Model file for the job. Use its own axes, mm. Coordinates: 2 decimals unless noted, no trailing zeros. Write each loop counter-clockwise with the first axis right and the second up, starting at its lowest first coordinate (ties: lowest second). Pieces come first, ordered by that corner, then holes. Notation, with made-up numbers: M 27,52 L 74,52 A33 cw 74,80 Z; hole C -35.5,12 d5. An arc over 180 degrees is marked long. Use CSV: the item, a comma, the result in double quotes. Start each with the question number.
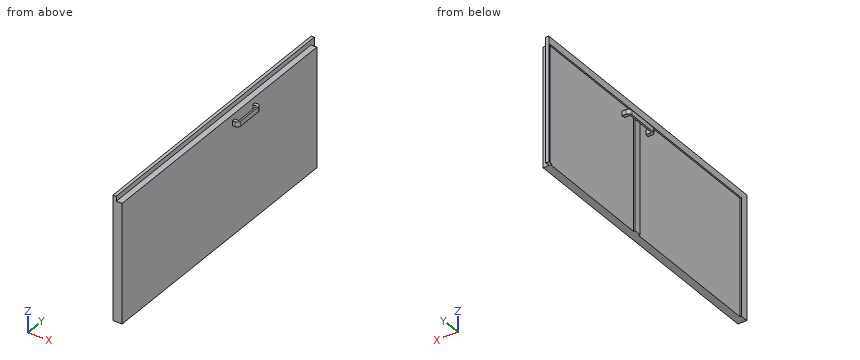
from build123d import *

# Parameters (mm, degrees)
SKETCH1_W            = 54.758446478
SKETCH1_H            = 717
BOSS_EXTRUDE1_DEPTH  = 1725
SKETCH2_W            = 19.21757675
SKETCH2_H            = 1725
BOSS_EXTRUDE2_DEPTH  = 30
SKETCH3_W            = 19.21757675
SKETCH3_H            = 747.470855808
BOSS_EXTRUDE3_DEPTH  = 30
SKETCH5_W            = 704.182305872
SKETCH5_H            = 1697.425748722
CUT_EXTRUDE1_DEPTH   = 8.60534571
SKETCH6_W            = 704.182305872
SKETCH6_H            = 43.914333375
BOSS_EXTRUDE5_DEPTH  = 9
SKETCH7_W            = 29.914870165
SKETCH7_H            = 20.630944942
BOSS_EXTRUDE6_DEPTH  = 35
SKETCH8_W            = 29.914870164
SKETCH8_H            = 20.630944941
BOSS_EXTRUDE7_DEPTH  = 35
SKETCH9_W            = 27.336002047
SKETCH9_H            = 231.066583342
BOSS_EXTRUDE8_DEPTH  = 10
SKETCH10_W           = 2.578868118
SKETCH10_H           = 20.630944942
CUT_EXTRUDE2_DEPTH   = 35
SKETCH11_W           = 2.578868117
SKETCH11_H           = 20.630944941
CUT_EXTRUDE3_DEPTH   = 35
FILLET2_R            = 20
FILLET3_R            = 20
SKETCH12_W           = 29.76753668
SKETCH12_H           = 18.691243962
SKETCH12_H_2         = 20.075780552
BOSS_EXTRUDE9_DEPTH  = 25
SKETCH13_W           = 29.76753668
SKETCH13_H           = 198.681000631
BOSS_EXTRUDE10_DEPTH = 10
FILLET4_R            = 20
FILLET5_R            = 20


with BuildPart() as part:
    # Sketch1 → Boss-Extrude1 (new body)
    with BuildSketch(Plane(origin=(0, 0, 0), x_dir=(1, 0, 0), z_dir=(0, 1, 0))):
        with Locations((27.379223239, -358.5)):
            Rectangle(SKETCH1_W, SKETCH1_H)
    extrude(amount=BOSS_EXTRUDE1_DEPTH)

    # Sketch2 → Boss-Extrude2 (add)
    with BuildSketch(Plane.XY.offset(717)):
        with Locations((9.608788375, 862.5)):
            Rectangle(SKETCH2_W, SKETCH2_H)
    extrude(amount=BOSS_EXTRUDE2_DEPTH)

    # Sketch3 → Boss-Extrude3 (add)
    with BuildSketch(Plane(origin=(0, 1725, 0), x_dir=(1, 0, 0), z_dir=(0, 1, 0))):
        with Locations((9.608788375, -373.264572096)):
            Rectangle(SKETCH3_W, SKETCH3_H)
    extrude(amount=BOSS_EXTRUDE3_DEPTH)

    # Sketch5 → Cut-Extrude1 (cut)
    with BuildSketch(Plane.ZY):
        with Locations((352.091152936, 896.687125639)):
            Rectangle(SKETCH5_W, SKETCH5_H)
    extrude(amount=-CUT_EXTRUDE1_DEPTH, mode=Mode.SUBTRACT)

    # Sketch6 → Boss-Extrude5 (add)
    with BuildSketch(Plane.ZY.offset(-8.60534571)):
        with Locations((352.091152936, 969.31583271)):
            Rectangle(SKETCH6_W, SKETCH6_H)
    extrude(amount=BOSS_EXTRUDE5_DEPTH)

    # Sketch7 → Boss-Extrude6 (add)
    with BuildSketch(Plane.ZY.offset(-8.60534571)):
        with Locations((647.577834423, 1083.33925491)):
            Rectangle(SKETCH7_W, SKETCH7_H)
    extrude(amount=BOSS_EXTRUDE6_DEPTH)

    # Sketch8 → Boss-Extrude7 (add)
    with BuildSketch(Plane.ZY.offset(-8.60534571)):
        with Locations((644.998966305, 872.90361651)):
            Rectangle(SKETCH8_W, SKETCH8_H)
    extrude(amount=BOSS_EXTRUDE7_DEPTH)

    # Sketch9 → Boss-Extrude8 (add)
    with BuildSketch(Plane.ZY.offset(26.39465429)):
        with Locations((646.288400364, 978.12143571)):
            Rectangle(SKETCH9_W, SKETCH9_H)
    extrude(amount=BOSS_EXTRUDE8_DEPTH)

    # Sketch10 → Cut-Extrude2 (cut)
    with BuildSketch(Plane.ZY.offset(26.39465429)):
        with Locations((661.245835446, 1083.33925491)):
            Rectangle(SKETCH10_W, SKETCH10_H)
    extrude(amount=-CUT_EXTRUDE2_DEPTH, mode=Mode.SUBTRACT)

    # Sketch11 → Cut-Extrude3 (cut)
    with BuildSketch(Plane.ZY.offset(26.39465429)):
        with Locations((631.330965282, 872.90361651)):
            Rectangle(SKETCH11_W, SKETCH11_H)
    extrude(amount=-CUT_EXTRUDE3_DEPTH, mode=Mode.SUBTRACT)

    # Fillet2
    fillet2_edges = [part.edges().sort_by_distance(p)[0] for p in [
        (-36.39465429, 862.588144039, 646.288400364),
    ]]
    fillet(fillet2_edges, radius=FILLET2_R)

    # Fillet3
    fillet3_edges = [part.edges().sort_by_distance(p)[0] for p in [
        (-36.39465429, 1093.654727381, 646.288400364),
    ]]
    fillet(fillet3_edges, radius=FILLET3_R)

    # Sketch12 → Boss-Extrude9 (add)
    with BuildSketch(Plane(origin=(54.758446478, 0, 0), x_dir=(0, 0, -1), z_dir=(1, 0, 0))):
        with Locations((-666.999193263, 1166.168231526)):
            Rectangle(SKETCH12_W, SKETCH12_H)
        with Locations((-666.999193263, 986.870743152)):
            Rectangle(SKETCH12_W, SKETCH12_H_2)
    extrude(amount=BOSS_EXTRUDE9_DEPTH)

    # Sketch13 → Boss-Extrude10 (add)
    with BuildSketch(Plane(origin=(79.758446478, 0, 0), x_dir=(0, 0, -1), z_dir=(1, 0, 0))):
        with Locations((-666.999193263, 1076.173353192)):
            Rectangle(SKETCH13_W, SKETCH13_H)
    extrude(amount=BOSS_EXTRUDE10_DEPTH)

    # Fillet4
    fillet4_edges = [part.edges().sort_by_distance(p)[0] for p in [
        (89.758446478, 1175.513853507, 666.999193263),
    ]]
    fillet(fillet4_edges, radius=FILLET4_R)

    # Fillet5
    fillet5_edges = [part.edges().sort_by_distance(p)[0] for p in [
        (89.758446478, 976.832852876, 666.999193263),
    ]]
    fillet(fillet5_edges, radius=FILLET5_R)


solid = part.part
1) Drop flat-ended pins along their axis: P1, Ø8, axis at y = 949, z = 651, coming from the +X side; P2, Ø10, axis at x = 29, y = 1308.5, coming from the -Z side; P3, Ø10.5, axis at x = 36.5, y = 1180.5, coming from the +Z side. Give the stop position or say it passes through.
2) Wall check: L1, parallel to Y at x = 4.5, z = 549; L2, parallel to X at y = 272, z = 515.5; L3, parallel to Y at x = 45, z = 477. Give the ranges that are in metal, low to high. Write a range as [from, to].
3) Band-saw the part on A-A on y = 1289. List the corners of the cut face in (x, z).
4) Band-saw the part on B-B on z = 263. List the corners of the cut face in (x, y), then the cut area to 3 significant figures.
Findings below:
1,P1,"stops at x = 54.76"
1,P2,"stops at z = 0"
1,P3,"stops at z = 717"
2,L1,"y = [0, 47.97], [947.36, 991.27], [1745.4, 1755]"
2,L2,"x = [8.61, 54.76]"
2,L3,"y = [0, 1725]"
3,outline,"M 0,704.18 L 8.61,704.18 L 8.61,0 L 54.76,0 L 54.76,717 L 19.22,717 L 19.22,747 L 0,747 Z"
4,outline,"M -0.39,947.36 L 8.61,947.36 L 8.61,47.97 L 0,47.97 L 0,0 L 54.76,0 L 54.76,1725 L 19.22,1725 L 19.22,1755 L 0,1755 L 0,1745.4 L 8.61,1745.4 L 8.61,991.27 L -0.39,991.27 Z"
4,area,"80,800 mm2"
